Can you work these out from the drawing? Everything is in mm from the part's minimum corner. A direction names the side the tool comes from. Round coordinates to 2 decimals unless told otherwise and drop trailing zeros. Order: outer loops, then holes, each group sorted by start corner. A loop starts at its lowest first (then second) coordinate and runs counter-clockwise, first axis right, second up. Notation, with made-up numbers: (-1, 78) - (50, 78) arc R14 ccw to (50, 93) - close; hole circle Ø2 at (19.5, 41.5). An arc over 180 degrees is marked (long way). Write item = value, one per line.
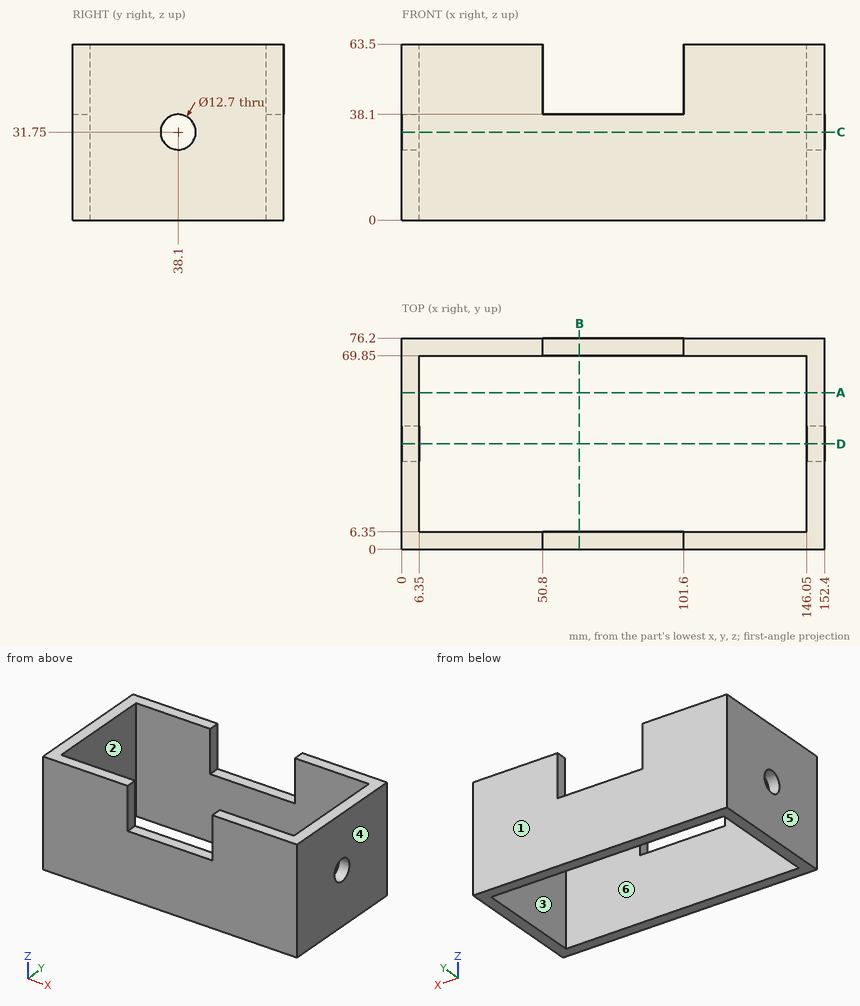
(1) Will these pins go through, and if not, where does the flat tip stop? P1, Ø1.9, axis at x = 83.5, y = 3.5, coming from the +Z side; P2, Ø8, axis at x = 58, y = 13.5, coming from the -Z side.
Computed:
P1 = 38.1
P2 = through
(2) Thinking about a two-plate mould opening in Y: for the marked faces 1, 2, 3 and 4, which applies, +Y half, -Y half, draft (parallel to the pull), parting line (faces both ways), or undercut?
Computed:
face_1 = +Y half
face_2 = undercut
face_3 = undercut
face_4 = draft
(3) If I drill on line 1 (Z direction, x = 2, y = 38.1); line 2 (X direction, y = 49.5, z = 26); line 3 (X direction, y = 71.5, z = 59.5), over which ranges is the centre line in solid material (lowest first)? Write a range as from..to.
Computed:
line_1 = 0..25.4, 38.1..63.5
line_2 = 0..6.35, 146.05..152.4
line_3 = 0..50.8, 101.6..152.4
(4) If we section it at D-D (y = 38.1): Write out the boundary of the cut face in (x, z), plus the area to 3 significant figures.
Computed:
outline = (0, 0) - (6.35, 0) - (6.35, 25.4) - (0, 25.4) - close; (0, 38.1) - (6.35, 38.1) - (6.35, 63.5) - (0, 63.5) - close; (146.05, 0) - (152.4, 0) - (152.4, 25.4) - (146.05, 25.4) - close; (146.05, 38.1) - (152.4, 38.1) - (152.4, 63.5) - (146.05, 63.5) - close
area = 645 mm^2
(5) If we section it at C-C (z = 31.75): Write out the boundary of the cut face in (x, y).
Computed:
outline = (0, 0) - (152.4, 0) - (152.4, 31.75) - (146.05, 31.75) - (146.05, 6.35) - (6.35, 6.35) - (6.35, 31.75) - (0, 31.75) - close; (0, 44.45) - (6.35, 44.45) - (6.35, 69.85) - (146.05, 69.85) - (146.05, 44.45) - (152.4, 44.45) - (152.4, 76.2) - (0, 76.2) - close
(6) If we section it at B-B (x = 64): Write out the boundary of the cut face in (y, z).
Computed:
outline = (0, 0) - (6.35, 0) - (6.35, 38.1) - (0, 38.1) - close; (69.85, 0) - (76.2, 0) - (76.2, 38.1) - (69.85, 38.1) - close
(7) On a 3-axis mill with a long thin cutter (end or side, diameter ignored), from which of +Z, -Z, +X, -X, +Y, -Y can I reach the whole of each face in a straight line? I mean the marked faces 5 and 6. Say none if no direction works.
Computed:
face_5 = +Z, -Z, -X, +Y, -Y
face_6 = +Z, -Z
(8) If we section it at A-A (y = 56.5): Write out the boundary of the cut face in (x, z), plus the area to 3 significant figures.
Computed:
outline = (0, 0) - (6.35, 0) - (6.35, 63.5) - (0, 63.5) - close; (146.05, 0) - (152.4, 0) - (152.4, 63.5) - (146.05, 63.5) - close
area = 806 mm^2
